```python
from build123d import *

# Parameters (mm, degrees)
EXTRUDE_THIN1_DEPTH = 508
FILLET1_R           = 1.27
FILLET2_R           = 0.889


with BuildPart() as part:
    # Sketch1 → Extrude-Thin1 (new body)
    with BuildSketch(Plane.XY):
        with BuildLine():
            Line((0, 44.45), (0, 50.8))
            ThreePointArc((0, 50.8), (-1.943679558, 50.278693106), (-2.794, 48.454794465))
            Line((-2.794, 48.454794465), (-2.794, 18.877476346))
            ThreePointArc((-2.794, 18.877476346), (-3.7465, 15.313547685), (-6.35, 12.7))
            Line((-6.35, 12.7), (-6.35, 0))
            Line((-6.35, 0), (-5.08, 0))
            Line((-5.08, 0), (-5.08, 12.007727151))
            ThreePointArc((-5.08, 12.007727151), (-2.465699307, 15.009705993), (-1.524, 18.877476346))
            Line((-1.524, 18.877476346), (-1.524, 48.454794465))
            ThreePointArc((-1.524, 48.454794465), (-1.458573987, 48.830465532), (-1.27, 49.161900539))
            Line((-1.27, 49.161900539), (-1.27, 44.45))
            Line((-1.27, 44.45), (0, 44.45))
        make_face()
    extrude(amount=-EXTRUDE_THIN1_DEPTH)

    # Fillet1
    fillet1_edges = [part.edges().sort_by_distance(p)[0] for p in [
        (-6.35, 12.7, -254),
    ]]
    fillet(fillet1_edges, radius=FILLET1_R)

    # Fillet2
    fillet2_edges = [part.edges().sort_by_distance(p)[0] for p in [
        (0, 50.8, -254),
    ]]
    fillet(fillet2_edges, radius=FILLET2_R)


solid = part.part
```
Read the model definition and answer for the solid it produces. Units are mm, in the model's axes. A direction names the side the tool comes from. Coordinates: 2 decimals unless noted, no trailing zeros. Loops run counter-clockwise (first coordinate to the right, second up) from the corner with the lowest first, then second, coordinate; pieces in that order, holes last. Notation, with made-up numbers: (49.25, 10.25) - (103.25, 10.25) arc R9 ccw to (103.25, 19.25) - close; hole circle Ø10 at (14, -35). An arc over 180 degrees is marked (long way). Answer in a Markdown table with one row per item.
1. Find section B-B, the plane y = 29. Write down the section's boundary in (x, z).
Conclusion:
| item | result |
|---|---|
| outline | (-2.79, -508) - (-1.52, -508) - (-1.52, 0) - (-2.79, 0) - close |
2. Find section A-A, the plane z = -182. Write down the section's boundary in (x, y), then the cut area to 3 significant figures.
Conclusion:
| item | result |
|---|---|
| outline | (-6.35, 0) - (-5.08, 0) - (-5.08, 12.01) arc R8.41 ccw to (-1.52, 18.88) - (-1.52, 48.45) arc R1.11 cw to (-1.27, 49.16) - (-1.27, 44.45) - (0, 44.45) - (0, 49.87) arc R0.89 ccw to (-1.17, 50.71) arc R2.38 ccw to (-2.79, 48.45) - (-2.79, 18.88) arc R7.14 cw to (-5.81, 13.04) arc R1.27 ccw to (-6.35, 12.01) - close |
| area | 73.2 mm² |
3. Straight lines are drawn through the part: line 1 (X direction, y = 8.5, z = -471); line 2 (X direction, y = 26, z = -40); line 3 (Y direction, x = -5.75, z = -165). For each, find the intervals that lie inside material, in ascending order.
Conclusion:
| item | result |
|---|---|
| line 1 | x = -6.35 to -5.08 |
| line 2 | x = -2.79 to -1.52 |
| line 3 | y = 0 to 13.09 |
4. Which of the six approach directions +Z, -Z, +X, -X, +Y, -Y give full straight-line access (tool end or side, diameter ignored) to faces 1 (the face through (-2.794, 34, -250)), 2 (the face through (-5.08, 6, -250)), 3 (the face through (-6.35, 6, -250))?
Conclusion:
| item | result |
|---|---|
| face 1 | +Z, -Z, -X, +Y |
| face 2 | +Z, -Z, +X, -Y |
| face 3 | +Z, -Z, -X, +Y, -Y |
5. Given pin 1 (15 mm diameter, centred on y = 27, z = -313.5, fed in from +X); pin 2 (6 mm diameter, centred on y = 39.5, z = -166.5, fed in from -X); pin 3 (1 mm diameter, centred on x = -0.5, z = -162, fed in from -Y), each flat-ended and moving along its own axis, determine where each tip first touches the part or whether it passes through.
Conclusion:
| item | result |
|---|---|
| pin 1 | stops at x = -1.52 |
| pin 2 | stops at x = -2.79 |
| pin 3 | stops at y = 44.45 |
